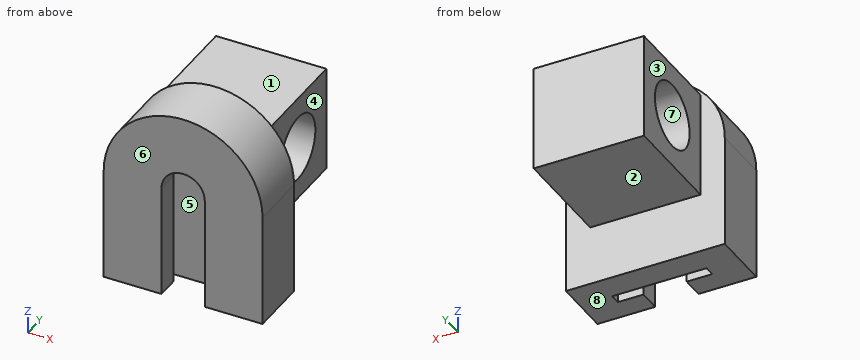
```python
from build123d import *

# Parameters (mm, degrees)
F1_DEPTH = 3.81
F3_DEPTH = 1.524
F5_DEPTH = 3.175
F6_W     = 15.875
F6_H     = 15.24
F7_DEPTH = 15.24
F8_R     = 4.6736
F9_DEPTH = 19.3685


with BuildPart() as f1:
    # F0 (on Front) → F1 (new body)
    with BuildSketch(Plane.XZ):
        with BuildLine():
            Line((-11.43, 0), (11.43, 0))
            ThreePointArc((11.43, 0), (0, 11.43), (-11.43, 0))
        make_face()
        with BuildLine():
            Line((11.43, -16.2387751043), (11.43, 0))
            ThreePointArc((11.43, 0), (0, -11.43), (-11.43, 0))
            Line((-11.43, 0), (-11.43, -16.2387751043))
            Line((-11.43, -16.2387751043), (11.43, -16.2387751043))
        make_face()
        with BuildLine():
            ThreePointArc((-11.43, 0), (0, -11.43), (11.43, 0))
            Line((11.43, 0), (-11.43, 0))
        make_face()
    extrude(amount=F1_DEPTH)

    # F2 (on face) → F3 (join)
    with BuildSketch(Plane.XZ.offset(3.81)):
        with BuildLine():
            Line((11.43, -16.2387751043), (11.43, 0))
            ThreePointArc((11.43, 0), (0, 11.43), (-11.43, 0))
            Line((-11.43, 0), (-11.43, -16.2387751043))
            Line((-11.43, -16.2387751043), (-6.7945, -16.2387751043))
            Line((-6.7945, -16.2387751043), (-6.7945, -11.6032751043))
            Line((-6.7945, -11.6032751043), (-6.7945, 0))
            ThreePointArc((-6.7945, 0), (0, 6.7945), (6.7945, 0))
            Line((6.7945, 0), (6.7945, -11.6032751043))
            Line((6.7945, -11.6032751043), (6.7945, -16.2387751043))
            Line((6.7945, -16.2387751043), (11.43, -16.2387751043))
        make_face()
    extrude(amount=F3_DEPTH)

    # F4 (on face) → F5 (join)
    with BuildSketch(Plane.XZ.offset(5.334)):
        with BuildLine():
            Line((-3.1115, -16.2387751043), (-3.1115, 0))
            ThreePointArc((-3.1115, 0), (0, 3.1115), (3.1115, 0))
            Line((3.1115, 0), (3.1115, -16.2387751043))
            Line((3.1115, -16.2387751043), (11.43, -16.2387751043))
            Line((11.43, -16.2387751043), (11.43, 0))
            ThreePointArc((11.43, 0), (0, 11.43), (-11.43, 0))
            Line((-11.43, 0), (-11.43, -16.2387751043))
            Line((-11.43, -16.2387751043), (-3.1115, -16.2387751043))
        make_face()
    extrude(amount=F5_DEPTH)

    # F6 (on face) → F7 (join)
    with BuildSketch(Plane(origin=(0, 0, 0), x_dir=(-1, 0, 0), z_dir=(0, 1, 0))):
        Rectangle(F6_W, F6_H)
    extrude(amount=F7_DEPTH)

    # F8 (on face) → F9 (cut, through all)
    with BuildSketch(Plane.YZ.offset(7.9375)):
        with Locations((7.62, 0)):
            Circle(F8_R)
    extrude(amount=-F9_DEPTH, mode=Mode.SUBTRACT)


solid = f1.part
```
The model under review builds one solid part; all positions refer to its coordinate system, in mm. Face numbers are marked on the shaded views. A direction names the side the tool comes from. Round coordinates to 2 decimals unless told otherwise and drop trailing zeros. Order: outer loops, then holes, each group sorted by start corner. A loop starts at its lowest first (then second) coordinate and runs counter-clockwise, first axis right, second up.
(1) Mouldability with a two-part tool opening along Y and no side actions: class the marked faces 6, 7 and 8 as released by +Y, released by -Y, zero draft, split by the parting line, or undercut.
Working result:
face 6: released by -Y
face 7: undercut
face 8: zero draft
(2) Wall thickness on L1, parallel to Z at x = 2, y = 7.62; L2, parallel to Y at x = -6.5, z = -13.25; L3, parallel to X at y = 14, z = -7: over which ranges is each line inside the solid? List them lowest first.
Working result:
L1: z = -7.62 to -4.67, 4.67 to 7.62
L2: y = -8.51 to -5.33, -3.81 to 0
L3: x = -7.94 to 7.94
(3) Take a section at C-C, the plane x = 7.25. State the section outline as (y, z) points.
Working result:
outline: (-8.51, -16.24) - (0, -16.24) - (0, -7.62) - (15.24, -7.62) - (15.24, 7.62) - (0, 7.62) - (0, 8.84) - (-8.51, 8.84) - close; hole circle Ø9.35 at (7.62, 0)
(4) Take a section at A-A, the plane z = 4. State the section outline as (x, y) points, plus the area to 3 significant figures.
Working result:
outline: (-10.71, -8.51) - (10.71, -8.51) - (10.71, 0) - (7.94, 0) - (7.94, 5.2) - (-7.94, 5.2) - (-7.94, 0) - (-10.71, 0) - close; (-7.94, 10.04) - (7.94, 10.04) - (7.94, 15.24) - (-7.94, 15.24) - close; hole (-5.49, -5.33) - (5.49, -5.33) - (5.49, -3.81) - (-5.49, -3.81) - close
area: 331 mm2
(5) Take a section at B-B, the plane y = 7.62. State the section outline as (x, z) points.
Working result:
outline: (-7.94, -7.62) - (7.94, -7.62) - (7.94, -4.67) - (-7.94, -4.67) - close; (-7.94, 4.67) - (7.94, 4.67) - (7.94, 7.62) - (-7.94, 7.62) - close
(6) For P1, Ø12, axis at y = 4.5, z = -1.5, coming from the -X side; P2, Ø3, axis at y = 2.5, z = -5.5, coming from the -X side; P3, Ø7.5, axis at x = 0, y = 6.5, coming from the +Z side; P4, Ø12, axis at y = 7.62, z = 0, coming from the +X side, all flat-tipped, find the tip position at first contact; note any pin that passes through.
Working result:
P1: stops at x = -11.43
P2: stops at x = -7.94
P3: stops at z = 7.62
P4: stops at x = 7.94
(7) Tool access review of the marked faces 1, 2, 3, 4 and 5: name each direction out of +Z, -Z, +X, -X, +Y, -Y from which nothing blocks a thin tool from reaching the whole face with its end or side.
Working result:
face 1: +Z, +X, -X, +Y
face 2: -Z, +X, -X, +Y
face 3: +Z, -Z, -X, +Y
face 4: +Z, -Z, +X, +Y
face 5: -Z
(8) Take a section at D-D, the plane z = -1.5. State the section outline as (x, y) points.
Working result:
outline: (-11.43, -8.51) - (-3.11, -8.51) - (-3.11, -5.33) - (-6.79, -5.33) - (-6.79, -3.81) - (6.79, -3.81) - (6.79, -5.33) - (3.11, -5.33) - (3.11, -8.51) - (11.43, -8.51) - (11.43, 0) - (7.94, 0) - (7.94, 3.19) - (-7.94, 3.19) - (-7.94, 0) - (-11.43, 0) - close; (-7.94, 12.05) - (7.94, 12.05) - (7.94, 15.24) - (-7.94, 15.24) - close
